Source: CAD feature listing. Evaluate the final solid. Frame: model axes, mm. A direction names the side the tool comes from. Give positions to 0.01 mm unless a question says otherwise; leave off trailing zeros. Loops run counter-clockwise (first coordinate to the right, second up) from the corner with the lowest first, then second, coordinate; pieces in that order, holes last. Notation, with made-up numbers: (14.25, 54) -> (38.25, 54) arc R24 cw to (38.25, 85) -> close; hole circle Ø1 at (4.5, -15). An arc over 180 degrees is marked (long way). Return JSON: item names as keys, results as strings. Group by question number.
```python
from build123d import *


with BuildPart() as part:
    # Sketch1 → Revolve1 (revolve)
    with BuildSketch(Plane.XY, mode=Mode.PRIVATE) as revolve1_sk:
        Polygon((0, 0), (140, 0), (140, -28.863803247), (136, -28.863803247), (136, -36.863803247), (140, -36.863803247), (140, -39.863803247), (136, -39.863803247), (136, -47.863803247), (140, -47.863803247), (140, -50.863803247), (136, -50.863803247), (136, -58.863803247), (140, -58.863803247), (140, -160), (130, -160), (130, -10), (0, -10), align=None)
    revolve(revolve1_sk.sketch.rotate(Axis((0, 0, 0), (0, -1, 0)), 90), axis=Axis((0, 0, 0), (0, -1, 0)))

    # Sketch2 → Revolve2 (revolve)
    with BuildSketch(Plane.XY, mode=Mode.PRIVATE) as revolve2_sk:
        with BuildLine():
            Line((0, 0), (0, -140))
            ThreePointArc((0, -140), (7.071067812, -142.928932188), (10, -150))
            Line((10, -150), (24, -150))
            Line((24, -150), (24, 0))
            Line((24, 0), (0, 0))
        make_face()
    revolve(revolve2_sk.sketch.rotate(Axis((0, 0, 0), (0, -1, 0)), 180), axis=Axis((0, 0, 0), (0, -1, 0)))


solid = part.part
```
1) Cut plane A-A on y = -108.5. Return loops of the section in (x, z), then the cut area to 3 significant figures.
2) Material intervals for line 1 (Y direction, x = -122.5, z = 67); line 2 (Z direction, x = 1.5, y = -126); line 3 (Z direction, x = -5.5, y = -28.5), sorted ascending.
3) Reachability of faces 4 (the face through (136.67, -110.14, -30.35)), 5 (the face through (-73, -50.864, -115)), 6 (the face through (-2, -10, 27)) from +Z, -Z, +X, -X, +Y, -Y: full face, straight path, thin tool, end or side. Return the list, or none.
4) Mould query, pull axis Y, two halves, no side actions, for faces 1 (the face through (-134.843, -54.92, -17.704)), 2 (the face through (124, -160, 41)), 3 (the face through (136.67, -14.63, -30.35)). Classes: released by +Y, released by -Y, zero draft, split by the parting line, or undercut.
5) Contact query for flat-ended pins moving along their axis: P1, Ø8, axis at x = -109.5, y = -119.5, coming from the -Z side; P2, Ø14.5, axis at x = -7, z = -11.5, coming from the -Y side; P3, Ø8, axis at y = -31, z = -46.5, coming from the -X side. Output: stop coordinate, or through.
Calculated:
{
 "1": {"outline": "circle Ø280 at (0, 0); circle Ø48 at (0, 0); hole circle Ø260 at (0, 0)", "area": "10,300 mm2"},
 "2": {"line 1": "-160 to -58.86, -50.86 to -47.86, -39.86 to -36.86, -28.86 to 0", "line 2": "-139.99 to -129.99, -23.95 to 23.95, 129.99 to 139.99", "line 3": "-139.89 to -129.88, -23.36 to 23.36, 129.88 to 139.89"},
 "3": {"face 4": "+Y, -Y", "face 5": "none", "face 6": "-Y"},
 "4": {"face 1": "undercut", "face 2": "released by -Y", "face 3": "zero draft"},
 "5": {"P1": "z = -92.03", "P2": "y = -150", "P3": "x = -133.19"}
}
